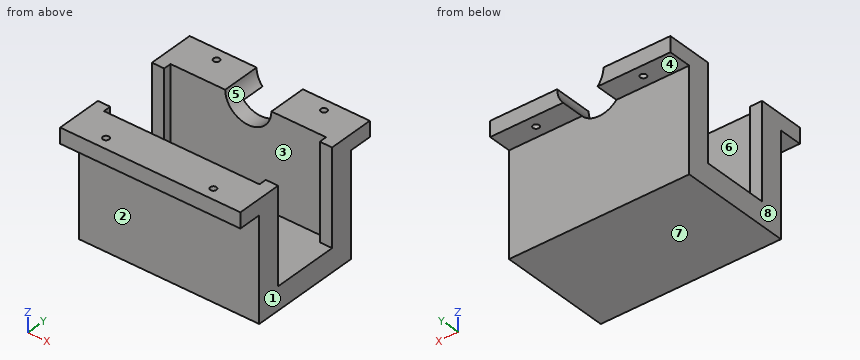
from build123d import *

# Parameters (mm, degrees)
F1_DEPTH  = 58.5
F3_DEPTH  = 136.4
F4_R      = 2
F5_DEPTH  = 25
F6_W      = 5
F6_H      = 31
F7_DEPTH  = 50.5
F8_W      = 117
F8_H      = 73
F9_DEPTH  = 31
F11_DEPTH = 31


with BuildPart() as f1:
    # F0 (on Right) → F1 (new body, symmetric)
    with BuildSketch(Plane.YZ):
        Polygon((51.5, 23), (36.5, 23), (21.5, 23), (21.5, -8), (0, -8), (-21.5, -8), (-21.5, 23), (-36.5, 23), (-51.5, 23), (-51.5, 13), (-36.5, 13), (-36.5, -23), (36.5, -23), (36.5, 13), (51.5, 13), align=None)
    extrude(amount=F1_DEPTH, both=True)

    # F2 (on Front) → F3 (cut)
    with BuildSketch(Plane.XZ):
        with BuildLine():
            ThreePointArc((-15, 23), (0, 8), (15, 23))
            Line((15, 23), (-15, 23))
        make_face()
    extrude(amount=-F3_DEPTH, mode=Mode.SUBTRACT)

    # F4 (on Top) → F5 (cut)
    with BuildSketch(Plane.XY):
        with Locations((-34.84017, -44)):
            Circle(F4_R)
        with Locations((34.84017, -44)):
            Circle(F4_R)
        with Locations((-34.84017, 44)):
            Circle(F4_R)
        with Locations((34.84017, 44)):
            Circle(F4_R)
    extrude(amount=F5_DEPTH, mode=Mode.SUBTRACT)

    # F6 (on Right) → F7 (cut, symmetric)
    with BuildSketch(Plane.YZ):
        with Locations((-24, 7.5)):
            Rectangle(F6_W, F6_H)
        with Locations((24, 7.5)):
            Rectangle(F6_W, F6_H)
    extrude(amount=F7_DEPTH, both=True, mode=Mode.SUBTRACT)

    # F8 (on face) → F9 (join)
    with BuildSketch(Plane(origin=(0, 0, -23), x_dir=(1, 0, 0), z_dir=(0, 0, -1))):
        Rectangle(F8_W, F8_H)
    extrude(amount=F9_DEPTH)

    # F10 (on face) → F11 (cut)
    with BuildSketch(Plane.XY.offset(-8)):
        Polygon((-50.5, 21.5), (-58.5, 21.5), (-58.5, -21.5), (-50.5, -21.5), (-50.5, -26.5), (50.5, -26.5), (50.5, -21.5), (58.5, -21.5), (58.5, 21.5), (50.5, 21.5), (50.5, 26.5), (-50.5, 26.5), align=None)
    extrude(amount=-F11_DEPTH, mode=Mode.SUBTRACT)


solid = f1.part
Here's how the part is built. I have some questions about the finished solid (model axes, mm). Face numbers are marked on the shaded views. A direction names the side the tool comes from. Round coordinates to 2 decimals unless told otherwise and drop trailing zeros. Write each loop counter-clockwise with the first axis right and the second up, starting at its lowest first coordinate (ties: lowest second). Pieces come first, ordered by that corner, then holes.
1. I need wall thicknesses on L1, parallel to X at y = -44, z = 17.75; L2, parallel to Y at x = -51, z = -32.5; L3, parallel to Y at x = 40.5, z = 3. Which ranges of each line are inside material? Lowest first, please.
2. Suppose I cut it at D-D (x = -30). List the corners of the cut face in (y, z) for me, and give its area (4 significant figures).
3. If we mould it in two halves opening along Y, with no side actions, what happens to the marked faces 1, 2 and 3? For each: released by +Y, released by -Y, zero draft, split by the parting line, or undercut.
4. Suppose I cut it at C-C (y = -44). List the corners of the cut face in (x, z) for me, and give its area (3 significant figures).
5. Suppose I cut it at A-A (y = 44). List the corners of the cut face in (x, z) for me.
6. For the marked faces 4, 5, 6, 7 and 8, which set-ups out of +Z, -Z, +X, -X, +Y, -Y let a thin tool reach every point of the face, with its end or its side?
7. Will these pins go through, and if not, where does the flat tip stop? pin 1 Ø12 at (x, y) = (-26.5, -46) entering from -Z; pin 2 Ø12 at (x, z) = (-5, -4.5) entering from +Y; pin 3 Ø6 at (x, y) = (20, 14.5) entering from +Z; pin 4 Ø8 at (x, y) = (-1.5, 39.5) entering from -Z.
8. Suppose I cut it at B-B (z = 3). List the corners of the cut face in (x, y) for me, and give its area (3 significant figures).
Answer sheet:
1. L1: x = -58.5 to -36.84, -32.84 to 32.84, 36.84 to 58.5
1. L2: y = -36.5 to -21.5, 21.5 to 36.5
1. L3: y = -36.5 to -26.5, 26.5 to 36.5
2. outline: (-51.5, 13) - (-36.5, 13) - (-36.5, -54) - (36.5, -54) - (36.5, 13) - (51.5, 13) - (51.5, 23) - (26.5, 23) - (26.5, -39) - (-26.5, -39) - (-26.5, 23) - (-51.5, 23) - close
2. area: 2,635 mm2
3. face 1: zero draft
3. face 2: released by -Y
3. face 3: undercut
4. outline: (-58.5, 13) - (-36.84, 13) - (-36.84, 23) - (-58.5, 23) - close; (-32.84, 13) - (32.84, 13) - (32.84, 23) - (-32.84, 23) - close; (36.84, 13) - (58.5, 13) - (58.5, 23) - (36.84, 23) - close
4. area: 1,090 mm2
5. outline: (-58.5, 13) - (-36.84, 13) - (-36.84, 23) - (-58.5, 23) - close; (-32.84, 13) - (-11.18, 13) arc R15 cw to (-15, 23) - (-32.84, 23) - close; (11.18, 13) - (32.84, 13) - (32.84, 23) - (15, 23) arc R15 cw to start; (36.84, 13) - (58.5, 13) - (58.5, 23) - (36.84, 23) - close
6. face 4: -Z, +X, -X, +Y
6. face 5: +Z, +Y
6. face 6: +Z
6. face 7: -Z, +X, -X, +Y, -Y
6. face 8: +Z, -Z, -X, +Y, -Y
7. pin 1: stops at z = 13
7. pin 2: stops at y = 36.5
7. pin 3: stops at z = -39
7. pin 4: stops at z = -54
8. outline: (-58.5, -36.5) - (58.5, -36.5) - (58.5, -21.5) - (50.5, -21.5) - (50.5, -26.5) - (-50.5, -26.5) - (-50.5, -21.5) - (-58.5, -21.5) - close; (-58.5, 21.5) - (-50.5, 21.5) - (-50.5, 26.5) - (50.5, 26.5) - (50.5, 21.5) - (58.5, 21.5) - (58.5, 36.5) - (-58.5, 36.5) - close
8. area: 2,500 mm2
